Input: dimensioned drawing with shaded views. Units: mm. Origin: part minimum x, y, z. Give positions to 0.01 mm unless a question says otherwise; leave off trailing zeros. Write each loop counter-clockwise with the first axis right and the second up, starting at its lowest first coordinate (ties: lowest second). Pieces come first, ordered by that corner, then holes.
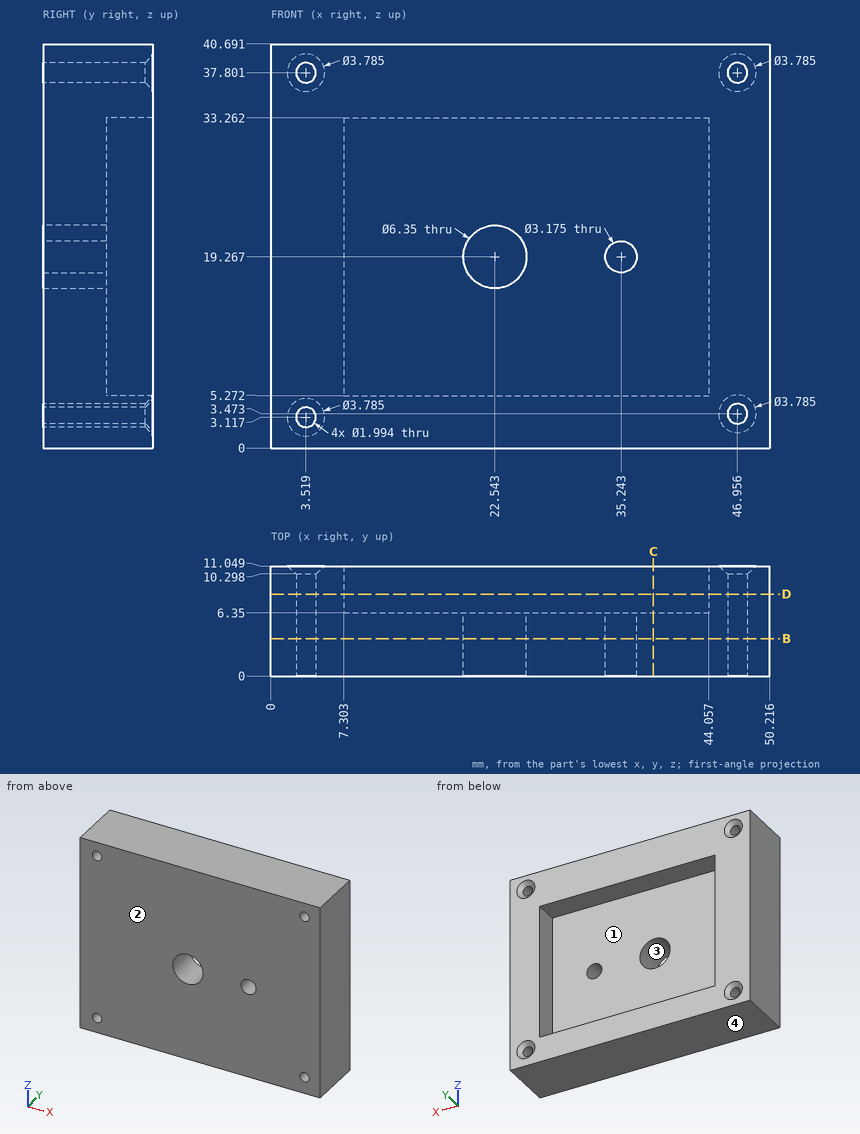
1. Cut plane C-C, the plane x = 38.5. Return the cut outline in (y, z), then the cut area to 3 significant figures.
2. Mould query, pull axis Z, two halves, no side actions, for the marked faces 1, 2, 3 and 4. Classes: +Z half, -Z half, draft (parallel to the pull), parting line (faces both ways), or undercut.
3. Cut plane D-D, the plane y = 8.25. Return the cut outline in (x, z) (1 decimal), then the cut area to 3 significant figures.
4. Line query: L1, parallel to X at y = 8.25, z = 32.5 (1 decimal); L2, parallel to Z at x = 29, y = 9; L3, parallel to X at y = 0.5, z = 19 (1 decimal). Output: solid intervals per line, ascending.
5. Cut plane B-B, the plane y = 3.75. State how many separate pieces and enclosed holes the cut face has, then the cut area to 3 significant figures.
6. Contact query for flat-ended pins moving along their axis: P1, Ø2.5, axis at x = 46.96, z = 37.8, coming from the +Y side (1 decimal); P2, Ø1.5, axis at x = 37, z = 20.5, coming from the +Y side. Output: stop coordinate, or through.
Response values:
1. outline: (0, 0) - (11.05, 0) - (11.05, 5.27) - (6.35, 5.27) - (6.35, 33.26) - (11.05, 33.26) - (11.05, 40.69) - (0, 40.69) - close
1. area: 318 mm2
2. face 1: undercut
2. face 2: draft
2. face 3: undercut
2. face 4: -Z half
3. outline: (0, 0) - (50.2, 0) - (50.2, 40.7) - (0, 40.7) - close; hole circle Ø2 at (3.5, 3.1); hole circle Ø2 at (3.5, 37.8); hole (7.3, 5.3) - (44.1, 5.3) - (44.1, 33.3) - (7.3, 33.3) - close; hole circle Ø2 at (47, 3.5); hole circle Ø2 at (47, 37.8)
3. area: 1,000 mm2
4. L1: x = 0 to 7.3, 44.1 to 50.2
4. L2: z = 0 to 5.27, 33.26 to 40.69
4. L3: x = 0 to 19.4, 25.7 to 33.7, 36.8 to 50.2
5. separate pieces: 1
5. enclosed holes: 6
5. area: 1,990 mm2
6. P1: stops at y = 10.5
6. P2: stops at y = 6.35
